```python
from build123d import *

# Parameters (mm, degrees)
SKETCH1_W           = 12.2
SKETCH1_H           = 23
BOSS_EXTRUDE1_DEPTH = 3
CUT_EXTRUDE2_DEPTH  = 4
SKETCH5_R           = 3.925
CUT_EXTRUDE3_DEPTH  = 4
SKETCH6_R           = 0.75
CUT_EXTRUDE4_DEPTH  = 4
SKETCH7_R           = 3.93
SKETCH7_R_2         = 0.75
CUT_EXTRUDE5_DEPTH  = 4
SKETCH8_R           = 0.75
CUT_EXTRUDE6_DEPTH  = 4


with BuildPart() as part:
    # Sketch1 → Boss-Extrude1 (new body)
    with BuildSketch(Plane.XY):
        with BuildLine():
            Line((22.600652844, 98.055778181), (24.552064, 100.123868682))
            ThreePointArc((24.552064, 100.123868682), (27.226414403, 102.085102355), (30.423169177, 102.967908395))
            Line((30.423169177, 102.967908395), (32.3981368, 102.967908395))
            Line((32.3981368, 102.967908395), (32.3981368, 97.967908395))
            Line((32.3981368, 97.967908395), (35.3981368, 97.967908395))
            Line((35.3981368, 97.967908395), (35.3981368, 102.967908395))
            Line((35.3981368, 102.967908395), (42.521983007, 102.967908395))
            ThreePointArc((42.521983007, 102.967908395), (45.313446231, 102.166024258), (47.714614303, 100.532109635))
            Line((47.714614303, 100.532109635), (51.351246918, 97.100651749))
            ThreePointArc((51.351246918, 97.100651749), (53.795711755, 95.446564433), (56.638770897, 94.65382999))
            Line((56.638770897, 94.65382999), (58.6881368, 94.65382999))
            Line((58.6881368, 94.65382999), (58.6881368, 89.65382999))
            Line((58.6881368, 89.65382999), (61.6881368, 89.65382999))
            Line((61.6881368, 89.65382999), (61.6881368, 94.65382999))
            Line((61.6881368, 94.65382999), (69.516671711, 94.65382999))
            ThreePointArc((69.516671711, 94.65382999), (72.270221934, 93.840698694), (74.140331494, 91.662187375))
            ThreePointArc((74.140331494, 91.662187375), (76.513167022, 88.89023599), (80.008265046, 87.842212737))
            Line((80.008265046, 87.842212737), (84.9781368, 87.921834161))
            Line((84.9781368, 87.921834161), (84.9781368, 82.921834161))
            Line((84.9781368, 82.921834161), (87.9781368, 82.921834161))
            Line((87.9781368, 82.921834161), (87.9781368, 87.921834161))
            Line((87.9781368, 87.921834161), (92.770707207, 87.921834161))
            ThreePointArc((92.770707207, 87.921834161), (96.955459046, 86.251143727), (98.839013483, 82.157786039))
            Line((98.839013483, 82.157786039), (93.399435569, 3.354416739))
            ThreePointArc((93.399435569, 3.354416739), (92.994237185, 1.145679097), (92.106398089, -0.916952583))
            Line((92.106398089, -0.916952583), (81.904303792, -18.77723742))
            ThreePointArc((81.904303792, -18.77723742), (80.072671375, -20.621586038), (77.562692027, -21.297235952))
            Line((77.562692027, -21.297235952), (70.304838359, -21.297235952))
            Line((70.304838359, -21.297235952), (70.304838359, 1.741579383))
            Line((70.304838359, 1.741579383), (67.304838359, 1.741579383))
            Line((67.304838359, 1.741579383), (67.304838359, -21.297235952))
            Line((67.304838359, -21.297235952), (64.304838359, -21.297235952))
            Line((64.304838359, -21.297235952), (64.304838359, 1.741579383))
            Line((64.304838359, 1.741579383), (61.304838359, 1.741579383))
            Line((61.304838359, 1.741579383), (61.304838359, -21.297235952))
            Line((61.304838359, -21.297235952), (31.304838359, -21.297235952))
            Line((31.304838359, -21.297235952), (31.304838359, 1.130887015))
            Line((31.304838359, 1.130887015), (28.304838359, 1.130887015))
            Line((28.304838359, 1.130887015), (28.304838359, -21.297235952))
            Line((28.304838359, -21.297235952), (25.304838359, -21.297235952))
            Line((25.304838359, -21.297235952), (25.304838359, 1.130887015))
            Line((25.304838359, 1.130887015), (22.304838359, 1.130887015))
            Line((22.304838359, 1.130887015), (22.304838359, -21.297235952))
            Line((22.304838359, -21.297235952), (13.483047429, -21.297235952))
            ThreePointArc((13.483047429, -21.297235952), (10.159531289, -20.032773458), (8.51699975, -16.878932137))
            Line((8.51699975, -16.878932137), (0, 10.609645279))
            Line((0, 10.609645279), (15.219519397, 16.399351506))
            Line((15.219519397, 16.399351506), (15.219519397, 20.261157087))
            Line((15.219519397, 20.261157087), (20.219519397, 20.261157087))
            Line((20.219519397, 20.261157087), (20.219519397, 25.341157087))
            Line((20.219519397, 25.341157087), (15.219519397, 25.341157087))
            Line((15.219519397, 25.341157087), (15.219519397, 32.909351506))
            Line((15.219519397, 32.909351506), (20.219519397, 32.909351506))
            Line((20.219519397, 32.909351506), (20.219519397, 37.989351506))
            Line((20.219519397, 37.989351506), (15.219519397, 37.989351506))
            Line((15.219519397, 37.989351506), (-2.165979283, 49.840454802))
            Line((-2.165979283, 49.840454802), (-5.425944103, 93.020454802))
            ThreePointArc((-5.425944103, 93.020454802), (-3.436216957, 95.650222165), (-0.241837421, 96.469142112))
            Line((-0.241837421, 96.469142112), (6.1081368, 96.487236066))
            Line((6.1081368, 96.487236066), (6.1081368, 91.487236066))
            Line((6.1081368, 91.487236066), (9.1081368, 91.487236066))
            Line((9.1081368, 91.487236066), (9.1081368, 96.487236066))
            Line((9.1081368, 96.487236066), (18.964020228, 96.487236066))
            ThreePointArc((18.964020228, 96.487236066), (20.944261448, 96.896087548), (22.600652844, 98.055778181))
        make_face()
        with Locations((81.8781368, 55.421834161)):
            Rectangle(SKETCH1_W, SKETCH1_H, mode=Mode.SUBTRACT)
        with Locations((55.5881368, 62.15382999)):
            Rectangle(SKETCH1_W, SKETCH1_H, mode=Mode.SUBTRACT)
        with Locations((29.2981368, 70.467908395)):
            Rectangle(SKETCH1_W, SKETCH1_H, mode=Mode.SUBTRACT)
        with Locations((15.2081368, 63.987236066)):
            Rectangle(SKETCH1_W, SKETCH1_H, mode=Mode.SUBTRACT)
    extrude(amount=BOSS_EXTRUDE1_DEPTH)

    # Sketch4 → Cut-Extrude2 (cut, through all)
    with BuildSketch(Plane(origin=(0, 0, 0), x_dir=(-1, 0, 0), z_dir=(0, 0, -1))):
        Polygon((-52.208167191, 44.022304868), (-29.701522137, 39.284063804), (-32.214850005, 27.345756427), (-54.72149506, 32.083997491), align=None)
    extrude(amount=-CUT_EXTRUDE2_DEPTH, mode=Mode.SUBTRACT)

    # Sketch5 → Cut-Extrude3 (cut, through all)
    with BuildSketch(Plane.XY.offset(3)):
        with Locations((15.2081368, 75.487236066)):
            Circle(SKETCH5_R)
        with Locations((29.2981368, 81.967908395)):
            Circle(SKETCH5_R)
        with Locations((55.5881368, 73.65382999)):
            Circle(SKETCH5_R)
        with Locations((81.8781368, 66.921834161)):
            Circle(SKETCH5_R)
    extrude(amount=-CUT_EXTRUDE3_DEPTH, mode=Mode.SUBTRACT)

    # Sketch6 → Cut-Extrude4 (cut, through all)
    with BuildSketch(Plane.XY.offset(3)):
        with Locations((15.2081368, 49.987236066)):
            Circle(SKETCH6_R)
        with Locations((29.2981368, 56.467908395)):
            Circle(SKETCH6_R)
        with Locations((55.5881368, 48.15382999)):
            Circle(SKETCH6_R)
        with Locations((81.8781368, 41.421834161)):
            Circle(SKETCH6_R)
    extrude(amount=-CUT_EXTRUDE4_DEPTH, mode=Mode.SUBTRACT)

    # Sketch7 → Cut-Extrude5 (cut, through all)
    with BuildSketch(Plane(origin=(0, 0, 0), x_dir=(-1, 0, 0), z_dir=(0, 0, -1))):
        with Locations((-30.958186071, 33.314910116)):
            Circle(SKETCH7_R)
        with Locations((-52.760024114, 36.18145487)):
            Circle(SKETCH7_R_2)
    extrude(amount=-CUT_EXTRUDE5_DEPTH, mode=Mode.SUBTRACT)

    # Sketch8 → Cut-Extrude6 (cut, through all)
    with BuildSketch(Plane.XY.offset(3)):
        with Locations((55.421930696, 38.465172142)):
            Circle(SKETCH8_R)
    extrude(amount=-CUT_EXTRUDE6_DEPTH, mode=Mode.SUBTRACT)


solid = part.part
```
Verification items for the finished model (mm, model axes). A direction names the side the tool comes from. Coordinates: 2 decimals unless noted, no trailing zeros. Write each loop counter-clockwise with the first axis right and the second up, starting at its lowest first coordinate (ties: lowest second). Pieces come first, ordered by that corner, then holes. Notation, with made-up numbers: (-37, -24) - (5, -24) arc R3 ccw to (5, -20) - close; hole circle Ø7 at (-5, 58). An arc over 180 degrees is marked (long way). One line per question, with ' | ' between items. Start each with the question number.
1. Draft check along X on faces 5 (the flat face through (87.978, 55, 1)), 6 (the cylindrical face through (53.758, 95.464, 1.479)), 7 (the flat face through (14, 96.487, 1)). Enter one of: released by +X, released by -X, zero draft, split by the parting line, or undercut.
2. Section check A-A (z = 1.5). Count the separate pieces of the cut face and the enclosed holes in it, plus the area to 3 significant figures.
3. Gauge pin test, flat ends, axial feed: P1, Ø1.5, axis at y = 84.5, z = 1, coming from the -X side; P2, Ø1.5, axis at y = 85, z = 2, coming from the +X side; P3, Ø1.5, axis at y = 54.5, z = 2, coming from the -X side. Record the tip position at first contact, or that the pin passes through.
4. Material ranges on line 1 along Y through (x, z) = (30.5, 0.65); line 2 along X through (y, z) = (0, 1.9); line 3 along X through (y, z) = (65.5, 1.1), recorded low to high.
5. Section check B-B (y = 6). Enter the section's corners in (x, z).
6. Access from +Z, -Z, +X, -X, +Y, -Y to the whole of each face (thin tool, end or side, straight path). Record for faces 1 (the flat face through (18, 32.909, 1)), 2 (the cylindrical face through (80.104, -20.603, 1.479)), 3 (the flat face through (23.198, 70, 1)), 4 (the flat face through (61.688, 92, 1)).
Computed values:
1) face 5: undercut | face 6: released by +X | face 7: zero draft
2) separate pieces: 1 | enclosed holes: 10 | area: 8,700 mm²
3) P1: x = -4.84 | P2: x = 98.35 | P3: x = -2.57
4) line 1: 1.13 to 29.41, 39.45 to 58.97, 85.7 to 102.97 | line 2: 3.29 to 22.3, 25.3 to 28.3, 31.3 to 61.3, 64.3 to 67.3, 70.3 to 92.57 | line 3: -3.35 to 9.11, 21.31 to 23.2, 35.4 to 49.49, 61.69 to 75.78, 87.98 to 97.69
5) outline: (1.43, 0) - (93.58, 0) - (93.58, 3) - (1.43, 3) - close
6) face 1: +Z, -Z, -X | face 2: +Z, -Z, +X, -Y | face 3: +Z, -Z | face 4: +Z, -Z, +Y
